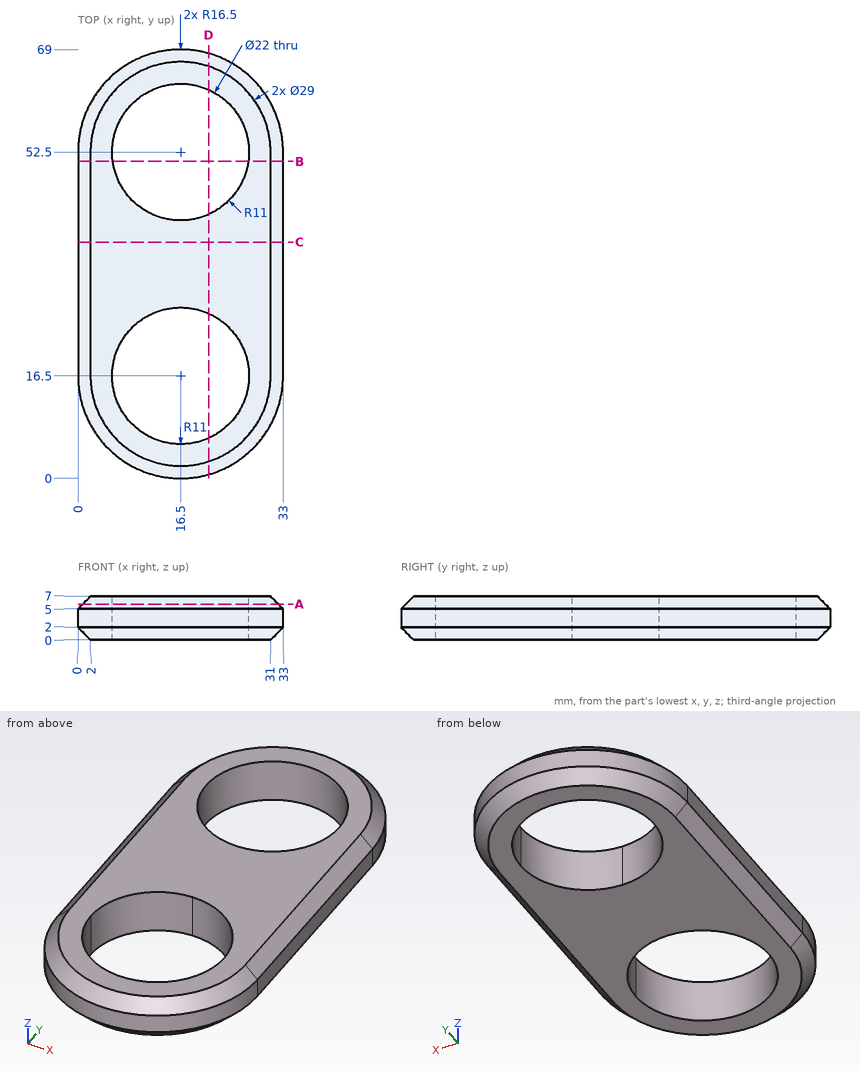
Answer from the drawing. Dimensions are ordinates in mm from the lowest x, y and z of the part. Give positions to 0.01 mm unless a question says otherwise; leave off trailing zeros. Write each loop counter-clockwise with the first axis right and the second up, starting at its lowest first coordinate (ties: lowest second). Pieces come first, ordered by that corner, then holes.
1) Section A-A (z = 5.75) is taken. Write down the section's boundary in (x, y).
2) Find the intervals of material crossed by L1, parallel to Y at x = 16.5, z = 2.75; L2, parallel to Y at x = 13, z = 6.75; L3, parallel to X at y = 52.5, z = 3.25, in increasing order.
3) Given P1, Ø2, axis at x = 5, z = 4.5, coming from the +Y side; P2, Ø1.5, axis at y = 57.5, z = 4.5, coming from the -X side, each flat-ended and moving along its own axis, determine where each tip first touches the part or whether it passes through.
4) Section C-C (y = 38) is taken. Write down the section's boundary in (x, z).
5) Section B-B (y = 51) is taken. Write down the section's boundary in (x, z).
6) Section D-D (x = 21) is taken. Count the separate pieces of the cut face and the enclosed holes in it, and give its area (3 significant figures).
Response:
1. outline: (0.75, 16.5) arc R15.75 ccw to (32.25, 16.5) - (32.25, 52.5) arc R15.75 ccw to (0.75, 52.5) - close; hole circle Ø22 at (16.5, 16.5); hole circle Ø22 at (16.5, 52.5)
2. L1: y = 0 to 5.5, 27.5 to 41.5, 63.5 to 69
2. L2: y = 2.17 to 6.07, 26.93 to 42.07, 62.93 to 66.83
2. L3: x = 0 to 5.5, 27.5 to 33
3. P1: stops at y = 65.23
3. P2: stops at x = 0.56
4. outline: (0, 2) - (2, 0) - (31, 0) - (33, 2) - (33, 5) - (31, 7) - (2, 7) - (0, 5) - close
5. outline: (0, 2) - (2, 0) - (5.6, 0) - (5.6, 7) - (2, 7) - (0, 5) - close; (27.4, 0) - (31, 0) - (33, 2) - (33, 5) - (31, 7) - (27.4, 7) - close
6. separate pieces: 3
6. enclosed holes: 0
6. area: 185 mm2
